Work out the finished part from the listing and answer in its coordinate system (mm). Coordinates: 2 decimals unless noted, no trailing zeros. Order: outer loops, then holes, each group sorted by start corner. A loop starts at its lowest first (then second) coordinate and runs counter-clockwise, first axis right, second up.
1. Determine the mould class of faces 1 (the cylindrical face through (-6.91, -4.04, -0.3)), 2 (the flat face through (2, -8, 8)), 3 (the flat face through (5.92, -3.94, 10.44)), 4 (the flat face through (-5.92, -3.94, -10.44)) for opening direction Z: +Z half, -Z half, draft (parallel to the pull), parting line (faces both ways), or undercut.
2. Find the intervals of material crossed by probe 1 along X at (y, z) = (-5.4, 0); probe 2 along X at (y, z) = (-2.25, 6.25); probe 3 along Z at (x, y) = (-0.25, -0.75), in increasing order.
3. The part is cut by section B-B, the plane z = 0. Give the vertices of the cut face in (x, y), then the cut area to 3 significant figures.
4. Flat-ended cylindrical pins translate along their axes: pin 1 Ø1 at (x, z) = (-5, -1.5) entering from +Y; pin 2 Ø1 at (x, y) = (-3.5, -2.5) entering from -Z; pin 3 Ø8 at (x, z) = (-7, -4.5) entering from +Y. Find the tip coordinate at first contact, or state that the pin passes through.
5. The part is cut by section A-A, the plane y = -5.75. Give the vertices of the cut face in (x, z) (1 decimal), then the cut area to 4 significant figures.
```python
from build123d import *

# Parameters (mm, degrees)
SKETCH2_W               = 96
SKETCH2_H               = 96
CUT_EXTRUDE1_DEPTH      = 9
CUT_EXTRUDE1_DEPTH_BACK = 9


with BuildPart() as part:
    # Sketch1 → Revolve1 (revolve)
    with BuildSketch(Plane.XY):
        Polygon((0, 0), (11.95, 0), (26.87820323, -4), (11.95, -8), (0, -8), align=None)
    revolve(axis=Axis((0, -8, 0), (0, 1, 0)))

    # Sketch2 → Cut-Extrude1 (cut, two sides)
    with BuildSketch(Plane(origin=(0, 0, 0), x_dir=(1, 0, 0), z_dir=(0, 1, 0))) as cut_extrude1_sk:
        Rectangle(SKETCH2_W, SKETCH2_H)
        Polygon((-12, -6.92820323), (0, -13.856406461), (12, -6.92820323), (12, 6.92820323), (0, 13.856406461), (-12, 6.92820323), align=None, mode=Mode.SUBTRACT)
    extrude(amount=CUT_EXTRUDE1_DEPTH, mode=Mode.SUBTRACT)
    extrude(cut_extrude1_sk.sketch, amount=-CUT_EXTRUDE1_DEPTH_BACK, mode=Mode.SUBTRACT)

    # Sketch3 → Cut-Revolve1 (revolve, cut)
    with BuildSketch(Plane.XY):
        Polygon((0, 0), (8, 0), (6.9175, -1.0825), (6.9175, -6.9175), (8, -8), (0, -8), align=None)
    revolve(axis=Axis((0, -8, 0), (0, 1, 0)), mode=Mode.SUBTRACT)


solid = part.part
```
Geometry says:
1. face 1: undercut
1. face 2: draft
1. face 3: +Z half
1. face 4: -Z half
2. probe 1: x = -12 to -6.92, 6.92 to 12
2. probe 2: x = -12 to -2.96, 2.96 to 12
2. probe 3: z = -13.71 to -7.25, 7.25 to 13.71
3. outline: (-12, -7.99) - (-11.95, -8) - (-8, -8) - (-6.92, -6.92) - (-6.92, -1.08) - (-8, 0) - (-11.95, 0) - (-12, -0.01) - close; (6.92, -6.92) - (8, -8) - (11.95, -8) - (12, -7.99) - (12, -0.01) - (11.95, 0) - (8, 0) - (6.92, -1.08) - close
3. area: 79.0 mm2
4. pin 1: passes through
4. pin 2: stops at z = -12.12
4. pin 3: stops at y = 0
5. outline: (-12, -6.9) - (0, -13.9) - (12, -6.9) - (12, 6.9) - (0, 13.9) - (-12, 6.9) - close; hole circle Ø13.8 at (0, 0)
5. area: 348.5 mm2
